```python
from build123d import *

# Parameters (mm, degrees)
SKETCH1_R           = 1
BOSS_EXTRUDE1_DEPTH = 2.3
CUT_EXTRUDE1_REACH  = 24.08
SKETCH2_R           = 1.5
SKETCH3_R           = 4.5
SKETCH3_R_2         = 2.25
BOSS_EXTRUDE2_DEPTH = 3


with BuildPart() as part:
    # Sketch1 → Boss-Extrude1 (new body)
    with BuildSketch(Plane.XY):
        with BuildLine():
            Line((-3.170292714, 6.987577235), (-1.469560928, 15.300650424))
            ThreePointArc((-1.469560928, 15.300650424), (0, 16.5), (1.469560928, 15.300650424))
            Line((1.469560928, 15.300650424), (3.170292714, 6.987577235))
            ThreePointArc((3.170292714, 6.987577235), (3.65, 6.321985448), (4.466273039, 6.239342646))
            Line((4.466273039, 6.239342646), (12.515971498, 8.923002309))
            ThreePointArc((12.515971498, 8.923002309), (14.289419162, 8.25), (13.985532426, 6.377648116))
            Line((13.985532426, 6.377648116), (7.636565754, 0.748234589))
            ThreePointArc((7.636565754, 0.748234589), (7.3, 0), (7.636565754, -0.748234589))
            Line((7.636565754, -0.748234589), (13.985532426, -6.377648116))
            ThreePointArc((13.985532426, -6.377648116), (14.289419162, -8.25), (12.515971498, -8.923002309))
            Line((12.515971498, -8.923002309), (4.466273039, -6.239342646))
            ThreePointArc((4.466273039, -6.239342646), (3.65, -6.321985448), (3.170292714, -6.987577235))
            Line((3.170292714, -6.987577235), (1.469560928, -15.300650424))
            ThreePointArc((1.469560928, -15.300650424), (0, -16.5), (-1.469560928, -15.300650424))
            Line((-1.469560928, -15.300650424), (-3.170292714, -6.987577235))
            ThreePointArc((-3.170292714, -6.987577235), (-3.65, -6.321985448), (-4.466273039, -6.239342646))
            Line((-4.466273039, -6.239342646), (-12.515971498, -8.923002309))
            ThreePointArc((-12.515971498, -8.923002309), (-14.289419162, -8.25), (-13.985532426, -6.377648116))
            Line((-13.985532426, -6.377648116), (-7.636565754, -0.748234589))
            ThreePointArc((-7.636565754, -0.748234589), (-7.3, 0), (-7.636565754, 0.748234589))
            Line((-7.636565754, 0.748234589), (-13.985532426, 6.377648116))
            ThreePointArc((-13.985532426, 6.377648116), (-14.289419162, 8.25), (-12.515971498, 8.923002309))
            Line((-12.515971498, 8.923002309), (-4.466273039, 6.239342646))
            ThreePointArc((-4.466273039, 6.239342646), (-3.65, 6.321985448), (-3.170292714, 6.987577235))
        make_face()
        with Locations((0, 14.2)):
            Circle(SKETCH1_R, mode=Mode.SUBTRACT)
        with Locations((0, 10.7)):
            Circle(SKETCH1_R, mode=Mode.SUBTRACT)
        with Locations((0, 7.2)):
            Circle(SKETCH1_R, mode=Mode.SUBTRACT)
        with Locations((6.235382907, 3.6)):
            Circle(SKETCH1_R, mode=Mode.SUBTRACT)
        with Locations((9.26647182, 5.35)):
            Circle(SKETCH1_R, mode=Mode.SUBTRACT)
        with Locations((12.297560734, 7.1)):
            Circle(SKETCH1_R, mode=Mode.SUBTRACT)
        with Locations((6.235382907, -3.6)):
            Circle(SKETCH1_R, mode=Mode.SUBTRACT)
        with Locations((9.26647182, -5.35)):
            Circle(SKETCH1_R, mode=Mode.SUBTRACT)
        with Locations((12.297560734, -7.1)):
            Circle(SKETCH1_R, mode=Mode.SUBTRACT)
        with Locations((0, -7.2)):
            Circle(SKETCH1_R, mode=Mode.SUBTRACT)
        with Locations((0, -10.7)):
            Circle(SKETCH1_R, mode=Mode.SUBTRACT)
        with Locations((0, -14.2)):
            Circle(SKETCH1_R, mode=Mode.SUBTRACT)
        with Locations((-6.235382907, -3.6)):
            Circle(SKETCH1_R, mode=Mode.SUBTRACT)
        with Locations((-9.26647182, -5.35)):
            Circle(SKETCH1_R, mode=Mode.SUBTRACT)
        with Locations((-12.297560734, -7.1)):
            Circle(SKETCH1_R, mode=Mode.SUBTRACT)
        with Locations((-6.235382907, 3.6)):
            Circle(SKETCH1_R, mode=Mode.SUBTRACT)
        with Locations((-9.26647182, 5.35)):
            Circle(SKETCH1_R, mode=Mode.SUBTRACT)
        with Locations((-12.297560734, 7.1)):
            Circle(SKETCH1_R, mode=Mode.SUBTRACT)
    extrude(amount=BOSS_EXTRUDE1_DEPTH)

    # Sketch2 → Cut-Extrude1 (cut, up to next)
    with BuildSketch(Plane.XY.offset(2.3), mode=Mode.PRIVATE) as cut_extrude1_sk1:
        Circle(SKETCH2_R)
    cut_extrude1_tool1 = extrude(cut_extrude1_sk1.sketch, amount=-CUT_EXTRUDE1_REACH, mode=Mode.PRIVATE) & part.part
    add(cut_extrude1_tool1.solids().sort_by_distance((0, 0, 2.3))[0], mode=Mode.SUBTRACT)

    # Sketch3 → Boss-Extrude2 (add)
    with BuildSketch(Plane.XY.offset(2.3)):
        Circle(SKETCH3_R)
        Circle(SKETCH3_R_2, mode=Mode.SUBTRACT)
    extrude(amount=BOSS_EXTRUDE2_DEPTH)


solid = part.part
```
Here's how the part is built. I have some questions about the finished solid (model axes, mm). A direction names the side the tool comes from. Round coordinates to 2 decimals unless told otherwise and drop trailing zeros. Order: outer loops, then holes, each group sorted by start corner. A loop starts at its lowest first (then second) coordinate and runs counter-clockwise, first axis right, second up. Notation, with made-up numbers: (-10.5, 67) -> (9.5, 67) arc R29 ccw to (9.5, 91) -> close; hole circle Ø8 at (46.5, 44.25). An arc over 180 degrees is marked (long way). Use a Markdown table: item, result. Add a question column.
(1) Suppose I cut it at B-B, the plane x = -9. Please give me the cut outline in (y, z).
(2) For pin 1 Ø1.6 at (x, y) = (0, 14.2) entering from +Z; pin 2 Ø2.5 at (x, y) = (0, 10.7) entering from +Z; pin 3 Ø1 at (x, z) = (8.5, 1) entering from +Y; pin 4 Ø2 at (x, z) = (-4, 4) entering from +Y, each with a flat end and sliding along its axis, tell me the tip position at first contact or that it passes through.
(3) If we mould it in two halves opening along Y, with no side actions, what happens to faces 1 (the face through (-2.33, 11.09, 1.13)), 2 (the face through (2.33, -11.09, 1.13)), 3 (the face through (8.473, -5.958, 1.134)), 4 (the face through (-10.855, -3.602, 1.134))? For each: released by +Y, released by -Y, zero draft, split by the parting line, or undercut.
(4) I need wall thicknesses on line 1 along Y through (x, z) = (12.5, 0.65); line 2 along Y through (x, z) = (7, 1.65); line 3 along X through (y, z) = (-5.5, 1.5). Which ranges of each line are inside material? Lowest first, please.
(5) Suppose I cut it at C-C, the plane y = 5.35. Please give me the cut outline in (x, z), and give its area (3 significant figures).
(6) Suppose I cut it at D-D, the plane z = 3.1. Please give me the cut outline in (x, y), and give its area (3 significant figures).
(7) Suppose I cut it at A-A, the plane y = -14.2. Please give me the cut outline in (x, z), and give its area (3 significant figures).
(8) For faces 5 (the face through (2.31, 11.2, 1.13)), 6 (the face through (-0.59, 4.46, 3.78)), 7 (the face through (-0.217, -11.676, 1.134)), which set-ups out of +Z, -Z, +X, -X, +Y, -Y let a thin tool reach every point of the face, with its end or its side?
Verdict:
| question | item | result |
|---|---|---|
| 1 | outline | (-7.75, 0) -> (-6.31, 0) -> (-6.31, 2.3) -> (-7.75, 2.3) -> close; (-4.39, 0) -> (-1.96, 0) -> (-1.96, 2.3) -> (-4.39, 2.3) -> close; (1.96, 0) -> (4.39, 0) -> (4.39, 2.3) -> (1.96, 2.3) -> close; (6.31, 0) -> (7.75, 0) -> (7.75, 2.3) -> (6.31, 2.3) -> close |
| 2 | pin 1 | through |
| 2 | pin 2 | z = 2.3 |
| 2 | pin 3 | y = 7.75 |
| 2 | pin 4 | y = 3.35 |
| 3 | face 1 | released by +Y |
| 3 | face 2 | released by -Y |
| 3 | face 3 | undercut |
| 3 | face 4 | undercut |
| 4 | line 1 | -8.92 to -8.08, -6.12 to -5.06, 5.06 to 6.12, 8.08 to 8.92 |
| 4 | line 2 | -7.08 to -4.24, -2.96 to 2.96, 4.24 to 7.08 |
| 4 | line 3 | -13 to -10.26, -8.28 to 8.28, 10.26 to 13 |
| 5 | outline | (-12.83, 0) -> (-10.27, 0) -> (-10.27, 2.3) -> (-12.83, 2.3) -> close; (-8.27, 0) -> (8.27, 0) -> (8.27, 2.3) -> (-8.27, 2.3) -> close; (10.27, 0) -> (12.83, 0) -> (12.83, 2.3) -> (10.27, 2.3) -> close |
| 5 | area | 49.8 mm2 |
| 6 | outline | circle Ø9 at (0, 0); hole circle Ø4.5 at (0, 0) |
| 6 | area | 47.7 mm2 |
| 7 | outline | (-1.69, 0) -> (-1, 0) -> (-1, 2.3) -> (-1.69, 2.3) -> close; (1, 0) -> (1.69, 0) -> (1.69, 2.3) -> (1, 2.3) -> close |
| 7 | area | 3.20 mm2 |
| 8 | face 5 | +Z, -Z, +Y |
| 8 | face 6 | +Z |
| 8 | face 7 | +Z, -Z |
